```python
from build123d import *

# Parameters (mm, degrees)
EXTRUDE_START       = -10
EXTRUDE_1_DEPTH     = 20
SKETCH_2_R          = 18
CUT_EXTRUDE_1_DEPTH = 159.773423469
SKETCH_3_R          = 10
CUT_EXTRUDE_2_DEPTH = 159.773423469
CUT_EXTRUDE_3_DEPTH = 6
CUT_EXTRUDE_4_DEPTH = 6
CHAMFER_1_SIZE      = 1
SKETCH_7_R          = 2
CUT_EXTRUDE_6_DEPTH = 25


# Read off the part's stored shape, not the designer's step: 凸台-拉伸1
with BuildPart() as part:
    # 凸台-拉伸1 outline → 凸台-拉伸1 (new body)
    with BuildSketch(Plane.XY.offset(EXTRUDE_START)):
        with BuildLine():
            ThreePointArc((2.6, 27.879024373), (-28, 0), (2.6, -27.879024373))
            Line((2.6, -27.879024373), (141.392857143, -14.935191628))
            ThreePointArc((141.392857143, -14.935191628), (155, 0), (141.392857143, 14.935191628))
            Line((141.392857143, 14.935191628), (2.6, 27.879024373))
        make_face()
    extrude(amount=EXTRUDE_1_DEPTH)

    # 草图2 → 切除-拉伸1 (cut, through all)
    with BuildSketch(Plane.XY.offset(10)):
        Circle(SKETCH_2_R)
    extrude(amount=-CUT_EXTRUDE_1_DEPTH, mode=Mode.SUBTRACT)

    # 草图3 → 切除-拉伸2 (cut, through all)
    with BuildSketch(Plane.XY.offset(10)):
        with Locations((140, 0)):
            Circle(SKETCH_3_R)
    extrude(amount=-CUT_EXTRUDE_2_DEPTH, mode=Mode.SUBTRACT)

    # 草图4 → 切除-拉伸3 (cut)
    with BuildSketch(Plane.XY.offset(10)):
        Polygon((40, -12), (40, 12), (110, 7), (110, -7), align=None)
    extrude(amount=-CUT_EXTRUDE_3_DEPTH, mode=Mode.SUBTRACT)

    # 草图5 → 切除-拉伸4 (cut)
    with BuildSketch(Plane.XY.offset(-10)):
        Polygon((40, -12), (40, 12), (110, 7), (110, -7), align=None)
    extrude(amount=CUT_EXTRUDE_4_DEPTH, mode=Mode.SUBTRACT)

    # 倒角1
    chamfer_1_edges = [part.edges().sort_by_distance(p)[0] for p in [
        (-18, 0, -10),
        (-18, 0, 10),
    ]]
    chamfer(chamfer_1_edges, length=CHAMFER_1_SIZE)

    # 草图7 → 切除-拉伸6 (cut)
    with BuildSketch(Plane(origin=(25, 0, 0), x_dir=(0, 0, -1), z_dir=(1, 0, 0))):
        Circle(SKETCH_7_R)
    extrude(amount=-CUT_EXTRUDE_6_DEPTH, mode=Mode.SUBTRACT)


solid = part.part
```
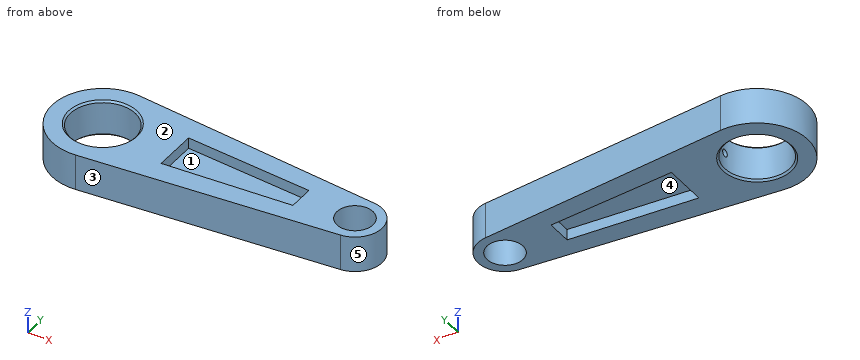
The model under review builds one solid part; all positions refer to its coordinate system, in mm. Face numbers are marked on the shaded views. A direction names the side the tool comes from. Round coordinates to 2 decimals unless told otherwise and drop trailing zeros. Write each loop counter-clockwise with the first axis right and the second up, starting at its lowest first coordinate (ties: lowest second). Pieces come first, ordered by that corner, then holes.
(1) Wall thickness on L1, parallel to X at y = -0.5, z = -3.5; L2, parallel to X at y = 1, z = 5.75; L3, parallel to X at y = 8, z = 3.25: over which ranges is each line inside the solid? List them lowest first.
(2) Machinability: for the marked faces 4 and 5, which of the approach directions +Z, -Z, +X, -X, +Y, -Y give a long, thin tool a straight path to every point of the face, cutting with its end or side? Answer none if there is none.
(3) We need section D-D on x = 58. Give the boundary of the cut face in (y, z).
(4) Mouldability with a two-part tool opening along X and no side actions: class the marked faces 1, 2 and 3 as +X half, -X half, draft (parallel to the pull), parting line (faces both ways), or undercut.
(5) We need section C-C on x = 0. Give the boundary of the cut face in (y, z), and give its area (3 significant figures).
(6) Insertion check: pin 1 (1.8 mm diameter, centred on y = -1.5, z = -6.5, fed in from -X); pin 2 (5 mm diameter, centred on y = 7.5, z = -2, fed in from -X); pin 3 (5 mm diameter, centred on y = -12.5, z = 1.5, fed in from +X). Each pin has a flat end and moves straight along its axis. Give the tip position at first contact, or say it passes through.
(7) We need section A-A on y = 0. Give the boundary of the cut face in (x, z).
(8) We need section B-B on z = 0. Give the boundary of the cut face in (x, y), and give its area (3 significant figures).
Findings below:
1. L1: x = -28 to -17.99, 17.99 to 130.01, 149.99 to 154.99
1. L2: x = -27.98 to -17.97, 17.97 to 40, 110 to 130.05, 149.95 to 154.97
1. L3: x = -26.83 to -16.12, 16.12 to 134, 146 to 152.69
2. face 4: -Z
2. face 5: +Z, -Z, +X
3. outline: (-22.71, -10) - (-10.71, -10) - (-10.71, -4) - (10.71, -4) - (10.71, -10) - (22.71, -10) - (22.71, 10) - (10.71, 10) - (10.71, 4) - (-10.71, 4) - (-10.71, 10) - (-22.71, 10) - close
4. face 1: undercut
4. face 2: draft
4. face 3: +X half
5. outline: (-28, -10) - (-19, -10) - (-18, -9) - (-18, 9) - (-19, 10) - (-28, 10) - close; (18, -9) - (19, -10) - (28, -10) - (28, 10) - (19, 10) - (18, 9) - close
5. area: 398 mm2
6. pin 1: stops at x = -27.99
6. pin 2: stops at x = -27.55
6. pin 3: stops at x = 151.18
7. outline: (-28, -10) - (-19, -10) - (-18, -9) - (-18, 9) - (-19, 10) - (-28, 10) - close; (18, -9) - (19, -10) - (40, -10) - (40, -4) - (110, -4) - (110, -10) - (130, -10) - (130, 10) - (110, 10) - (110, 4) - (40, 4) - (40, 10) - (19, 10) - (18, 9) - (18, 2) - (25, 2) - (25, -2) - (18, -2) - close; (150, -10) - (155, -10) - (155, 10) - (150, 10) - close
8. outline: (2.6, -27.88) - (141.39, -14.94) arc R15 ccw to (141.39, 14.94) - (2.6, 27.88) arc R28 ccw (long way) to start; hole (17.89, -2) - (25, -2) - (25, 2) - (17.89, 2) arc R18 ccw (long way) to start; hole circle Ø20 at (140, 0)
8. area: 6,270 mm2
